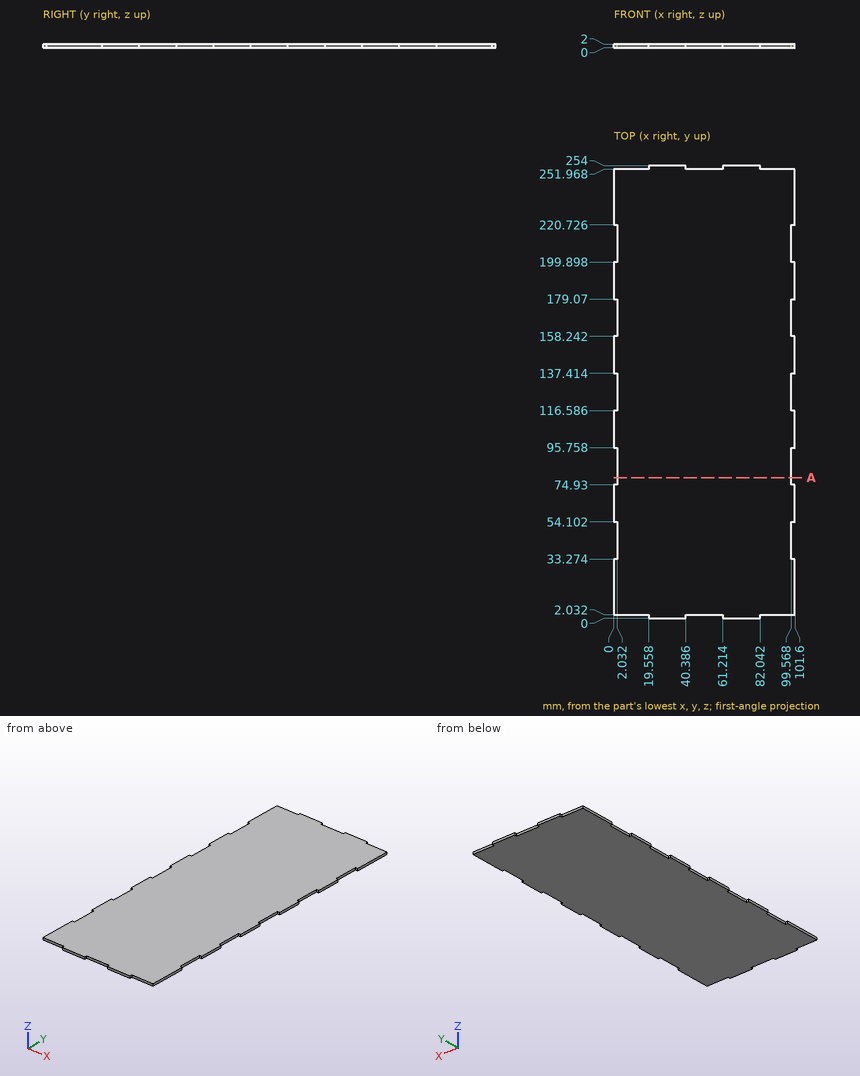
Answer from the drawing. Dimensions are ordinates in mm from the lowest x, y and z of the part. Round coordinates to 2 decimals unless told otherwise and drop trailing zeros. Order: outer loops, then holes, each group sorted by start corner. A loop starts at its lowest first (then second) coordinate and runs counter-clockwise, first axis right, second up.
1) The part is cut by section A-A on y = 79. Write down the section's boundary in (x, z), plus the area to 3 significant figures.
2) Flat-ended cylindrical pins translate along their axes: pin 1 (0.6 mm diameter, centred on x = 100, z = 1, fed in from -Y); pin 2 (1 mm diameter, centred on y = 1, z = 1, fed in from -X); pin 3 (0.6 mm diameter, centred on y = 252.5, z = 1.5, fed in from +X). Find the tip coordinate at first contact, or state that the pin passes through.
3) Straight lines are drawn through the part: L1, parallel to X at y = 80.5, z = 0.7; L2, parallel to Y at x = 51, z = 0.4. For each, find the intervals that lie inside material, in ascending order.
Resolved:
1. outline: (2.03, 0) - (99.57, 0) - (99.57, 2) - (2.03, 2) - close
1. area: 195 mm2
2. pin 1: stops at y = 2.03
2. pin 2: stops at x = 19.56
2. pin 3: stops at x = 82.04
3. L1: x = 2.03 to 99.57
3. L2: y = 2.03 to 251.97
